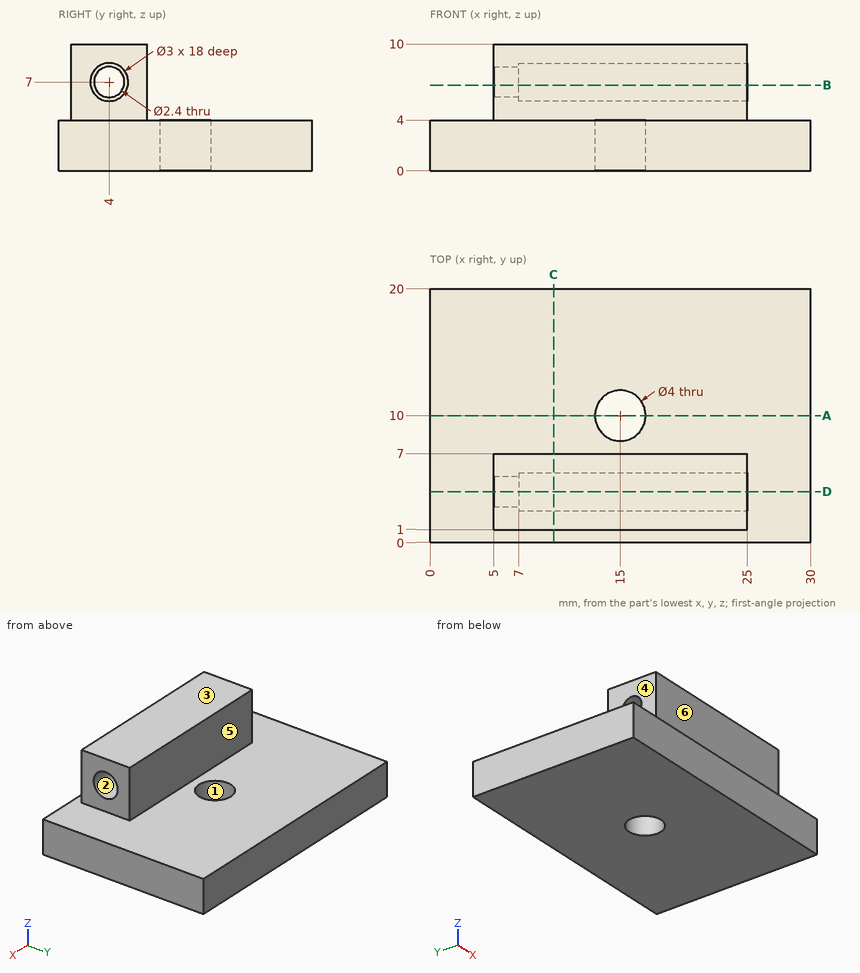
Here's the drawing with two shaded views (mm, measured from the low corner). I have some questions. A direction names the side the tool comes from. Coordinates: 2 decimals unless noted, no trailing zeros. Write each loop counter-clockwise with the first axis right and the second up, starting at its lowest first coordinate (ties: lowest second). Pieces come first, ordered by that corner, then holes.
Item 1: I want a section at D-D on y = 4. Write out the boundary of the cut face in (x, z), and give its area (3 significant figures).
Item 2: I want a section at C-C on x = 9.75. Write out the boundary of the cut face in (y, z).
Item 3: If we mould it in two halves opening along Z, with no side actions, what happens to the marked faces 1, 2 and 3? For each: +Z half, -Z half, draft (parallel to the pull), parting line (faces both ways), or undercut.
Item 4: On a 3-axis mill with a long thin cutter (end or side, diameter ignored), from which of +Z, -Z, +X, -X, +Y, -Y can I reach the whole of each face in a straight line? I mean the marked faces 4, 5 and 6. Say none if no direction works.
Item 5: I want a section at A-A on y = 10. Write out the boundary of the cut face in (x, z), and give its area (3 significant figures).
Item 6: I want a section at B-B on z = 6.75. Write out the boundary of the cut face in (x, y).
Item 7: Will these pins go through, and if not, where does the flat tip stop? pin 1 (5 mm diameter, centred on x = 15.5, z = 7.5, fed in from +Y); pin 2 (3 mm diameter, centred on x = 14, z = 7.5, fed in from -Y); pin 3 (3.5 mm diameter, centred on x = 15, y = 10, fed in from +Z); pin 4 (3 mm diameter, centred on y = 3, z = 6, fed in from -X).
Item 8: If I drill on line 1 (Y direction, x = 5.5, z = 7); line 2 (Y direction, x = 15, z = 1.9); line 3 (Y direction, x = 19.25, z = 4.5), over which ranges is the centre line in solid material (lowest first)?
Findings below:
1. outline: (0, 0) - (30, 0) - (30, 4) - (25, 4) - (25, 5.5) - (7, 5.5) - (7, 5.8) - (5, 5.8) - (5, 4) - (0, 4) - close; (5, 8.2) - (7, 8.2) - (7, 8.5) - (25, 8.5) - (25, 10) - (5, 10) - close
1. area: 181 mm2
2. outline: (0, 0) - (20, 0) - (20, 4) - (7, 4) - (7, 10) - (1, 10) - (1, 4) - (0, 4) - close; hole circle Ø3 at (4, 7)
3. face 1: draft
3. face 2: undercut
3. face 3: +Z half
4. face 4: +Z, -X, +Y, -Y
4. face 5: +Z, +X, -X, +Y
4. face 6: +Z, +X, -X, -Y
5. outline: (0, 0) - (13, 0) - (13, 4) - (0, 4) - close; (17, 0) - (30, 0) - (30, 4) - (17, 4) - close
5. area: 104 mm2
6. outline: (5, 1) - (25, 1) - (25, 2.52) - (7, 2.52) - (7, 2.83) - (5, 2.83) - close; (5, 5.17) - (7, 5.17) - (7, 5.48) - (25, 5.48) - (25, 7) - (5, 7) - close
7. pin 1: stops at y = 7
7. pin 2: stops at y = 1
7. pin 3: passes through
7. pin 4: stops at x = 5
8. line 1: y = 1 to 2.8, 5.2 to 7
8. line 2: y = 0 to 8, 12 to 20
8. line 3: y = 1 to 7
